The listing builds one solid part. Answer for the finished solid, in the listing's coordinates (mm). A direction names the side the tool comes from. Coordinates: 2 decimals unless noted, no trailing zeros. Order: outer loops, then holes, each group sorted by start corner. A loop starts at its lowest first (then second) coordinate and runs counter-clockwise, first axis right, second up. Notation, with made-up numbers: (48.5, 74.5) -> (52.5, 74.5) arc R18 cw to (52.5, 105.5) -> close; hole circle Ø4 at (40, 60). An arc over 180 degrees is marked (long way). Write each question's results on one line, items separated by ' | '. Start each with the question number.
(1) The part is cut by section B-B, the plane x = 9. Give the vertices of the cut face in (y, z), then the cut area to 3 significant figures.
(2) Straight lines are drawn through the part: L1, parallel to Z at x = 27.5, y = 7.25; L2, parallel to Y at x = 4, z = -26.5. For each, find the intervals that lie inside material, in ascending order.
(3) The part is cut by section C-C, the plane z = 21. Give the vertices of the cut face in (x, y), then the cut area to 3 significant figures.
(4) The part is cut by section A-A, the plane y = 7.75. Give the vertices of the cut face in (x, z), then the cut area to 3 significant figures.
(5) A tool of negligible diameter and unlimited length cuts with its end or side. For faces 4 (the face through (50, 5, 0)), 5 (the face through (25, 7, -25)), from which of +Z, -Z, +X, -X, +Y, -Y can it reach the whole face along a straight path? Write none if from no direction.
(6) Determine the mould class of faces 1 (the face through (25, 5, 35)), 2 (the face through (25, 10, 32)), 3 (the face through (25, 8, 20)) for opening direction Z: +Z half, -Z half, draft (parallel to the pull), parting line (faces both ways), or undercut.
(7) Given pin 1 (3 mm diameter, centred on x = 21, z = -23.5, fed in from +Y), flat-ended and moving along its own axis, determine where the tip first touches the part or whether it passes through.
```python
from build123d import *

# Parameters (mm, degrees)
SKETCH1_W           = 50
SKETCH1_H           = 70
BOSS_EXTRUDE1_DEPTH = 10
SKETCH3_W           = 10
SKETCH3_H           = 3
CUT_EXTRUDE1_DEPTH  = 62.846584384


with BuildPart() as part:
    # Sketch1 → Boss-Extrude1 (new body)
    with BuildSketch(Plane(origin=(0, 0, 0), x_dir=(1, 0, 0), z_dir=(0, 1, 0))):
        with Locations((25, 0)):
            Rectangle(SKETCH1_W, SKETCH1_H)
    extrude(amount=BOSS_EXTRUDE1_DEPTH)

    # Sketch3 → Cut-Extrude1 (cut, through all)
    with BuildSketch(Plane.ZY):
        with Locations((-25, 8.5)):
            Rectangle(SKETCH3_W, SKETCH3_H)
        with Locations((25, 8.5)):
            Rectangle(SKETCH3_W, SKETCH3_H)
    extrude(amount=-CUT_EXTRUDE1_DEPTH, mode=Mode.SUBTRACT)


solid = part.part
```
Established:
1) outline: (0, -35) -> (10, -35) -> (10, -30) -> (7, -30) -> (7, -20) -> (10, -20) -> (10, 20) -> (7, 20) -> (7, 30) -> (10, 30) -> (10, 35) -> (0, 35) -> close | area: 640 mm^2
2) L1: z = -35 to -30, -20 to 20, 30 to 35 | L2: y = 0 to 7
3) outline: (0, 0) -> (50, 0) -> (50, 7) -> (0, 7) -> close | area: 350 mm^2
4) outline: (0, -35) -> (50, -35) -> (50, -30) -> (0, -30) -> close; (0, -20) -> (50, -20) -> (50, 20) -> (0, 20) -> close; (0, 30) -> (50, 30) -> (50, 35) -> (0, 35) -> close | area: 2,500 mm^2
5) face 4: +Z, -Z, +X, +Y, -Y | face 5: +X, -X, +Y
6) face 1: +Z half | face 2: draft | face 3: undercut
7) pin 1: stops at y = 7
